Source: CAD feature listing. Evaluate the final solid. Frame: model axes, mm. A direction names the side the tool comes from. Give positions to 0.01 mm unless a question says otherwise; leave off trailing zeros. Write each loop counter-clockwise with the first axis right and the second up, starting at its lowest first coordinate (ties: lowest second). Pieces come first, ordered by that corner, then holes.
```python
from build123d import *

# Parameters (mm, degrees)
BOSS_EXTRUDE1_START = -30.1625
BOSS_EXTRUDE1_DEPTH = 60.325
CUT_EXTRUDE3_REACH  = 45.791
SKETCH2_W           = 60.325
SKETCH2_H           = 6.35
SKETCH3_W           = 1.5875
SKETCH3_H           = 16.002
CUT_EXTRUDE4_DEPTH  = 45.394636066


# Read off the part's stored shape, not the designer's step: Boss-Extrude1
with BuildPart() as part:
    # Boss-Extrude1 outline → Boss-Extrude1 (new body)
    with BuildSketch(Plane.YZ.offset(BOSS_EXTRUDE1_START)):
        Polygon((-1.5875, 33.25479651), (-1.5875, 0), (0, 0), (0, 31.384816574), align=None)
    extrude(amount=BOSS_EXTRUDE1_DEPTH)

    # Sketch2 → Cut-Extrude3 (cut, up to next)
    with BuildSketch(Plane(origin=(0, 18.958587107, 9.052736266), x_dir=(1, 0, 0), z_dir=(0, 0.7623380888196845, 0.6471789847752716)), mode=Mode.PRIVATE) as cut_extrude3_sk1:
        with Locations((0, -33.979180387)):
            Rectangle(SKETCH2_W, SKETCH2_H)
    cut_extrude3_tool1 = extrude(cut_extrude3_sk1.sketch, amount=-CUT_EXTRUDE3_REACH, mode=Mode.PRIVATE) & part.part
    add(cut_extrude3_tool1.solids().sort_by_distance((0, -3.032024, 34.95636))[0], mode=Mode.SUBTRACT)

    # Sketch3 → Cut-Extrude4 (cut, through all)
    with BuildSketch(Plane(origin=(0, 0, 0), x_dir=(1, 0, 0), z_dir=(0, 1, 0))):
        with Locations((29.36875, -15.70482)):
            Rectangle(SKETCH3_W, SKETCH3_H)
        with Locations((-29.36875, -15.70482)):
            Rectangle(SKETCH3_W, SKETCH3_H)
    extrude(amount=-CUT_EXTRUDE4_DEPTH, mode=Mode.SUBTRACT)


solid = part.part
```
1. Mould query, pull axis Z, two halves, no side actions, for faces 1 (the flat face through (28.575, -1, 16)), 2 (the flat face through (30.162, -1, 4)), 3 (the flat face through (-0.42, -0.48, 31.95)). Classes: +Z half, -Z half, draft (parallel to the pull), parting line (faces both ways), or undercut.
2. Cut plane A-A, the plane y = -0.7. Return the cut outline in (x, z) (1 decimal).
3. Cut plane B-B, the plane z = 19. Return the cut outline in (x, y) (1 decimal), then the cut area to 3 significant figures.
4. Contact query for flat-ended pins moving along their axis: P1, Ø0.5, axis at x = 29.5, y = -1, coming from the +Z side; P2, Ø0.8, axis at y = -1, z = 14.5, coming from the +X side (3 decimals). Output: stop coordinate, or through.
5. Line query: L1, parallel to X at y = -1.3, z = 20.5 (3 decimals); L2, parallel to Z at x = -5, y = -0.3; L3, parallel to Z at x = 19.5, y = -1.25. Output: solid intervals per line, ascending.
6. Access query for faces 4 (the flat face through (0, 0, 15)), 5 (the flat face through (29, -1, 7.704)), 6 (the flat face through (-29, -1, 23.706)). Directions: +Z, -Z, +X, -X, +Y, -Y. A direction counts if a zero-diameter tool reaches every point of the face in a straight line with its end or side. Return the directions, or none.
Response values:
1. face 1: undercut
1. face 2: draft
1. face 3: +Z half
2. outline: (-30.2, 0) - (30.2, 0) - (30.2, 7.7) - (28.6, 7.7) - (28.6, 23.7) - (30.2, 23.7) - (30.2, 32.2) - (-30.2, 32.2) - (-30.2, 23.7) - (-28.6, 23.7) - (-28.6, 7.7) - (-30.2, 7.7) - close
3. outline: (-28.6, -1.6) - (28.6, -1.6) - (28.6, 0) - (-28.6, 0) - close
3. area: 90.7 mm2
4. P1: stops at z = 32.54
4. P2: stops at x = 28.575
5. L1: x = -28.575 to 28.575
5. L2: z = 0 to 31.74
5. L3: z = 0 to 32.3
6. face 4: +Z, -Z, +X, -X, +Y
6. face 5: +X, +Y, -Y
6. face 6: -X, +Y, -Y
